Input: part model. Units: mm. Frame: model coordinates. A direction names the side the tool comes from. Round coordinates to 2 decimals unless told otherwise and drop trailing zeros. Loops run counter-clockwise (first coordinate to the right, second up) from the corner with the lowest first, then second, coordinate; pieces in that order, holes last. Notation, with made-up numbers: (16, -2) - (34, -2) arc R26 ccw to (34, 18) - close; hole circle Ø5 at (44, 14). An arc over 180 degrees is marked (long way). One line per question, with ' | ' between items. Start each with the question number.
Item 1: Set-up query: faces 4 (the face through (-7, 50, 25)), 5 (the face through (-380, 0, 25)). Return all of +Z, -Z, +X, -X, +Y, -Y with unobstructed straight access to the full face (end or side cutting, diameter ignored); none if empty.
Item 2: Material intervals for line 1 along Y through (x, z) = (60, 39); line 2 along Y through (x, z) = (-289.5, 4), sorted ascending.
Item 3: First-contact query: pin 1 (4 mm diameter, centred on x = -263, y = 16, fed in from -Z). Flat tip, straight axial feed; report the tip coordinate or a pass-through.
Item 4: Draft query along Y for faces 1 (the face through (-7, -50, 25)), 2 (the face through (-400, 10, 25)), 3 (the face through (-500, 1, 25)). Return one class per face: pulls with the +Y half, pulls with the -Y half, needs draft (parallel to the pull), parting line crosses it, or undercut.
Item 5: Section B-B, the plane y = 0. Give the number of separate pieces and of enclosed holes in the cut face, plus the area to 3 significant figures.
Item 6: Section A-A, the plane x = -392.5. Return loops of the section in (y, z), plus the area to 3 significant figures.
```python
from build123d import *

# Parameters (mm, degrees)
SKETCH1_W           = 900
SKETCH1_H           = 100
BOSS_EXTRUDE1_DEPTH = 50
SKETCH2_W           = 40
SKETCH2_H           = 20
CUT_EXTRUDE1_DEPTH  = 50
SKETCH3_W           = 50
SKETCH3_H           = 50
BOSS_EXTRUDE2_DEPTH = 100


with BuildPart() as part:
    # Sketch1 → Boss-Extrude1 (new body)
    with BuildSketch(Plane.XY):
        Rectangle(SKETCH1_W, SKETCH1_H)
    extrude(amount=BOSS_EXTRUDE1_DEPTH)

    # Sketch2 → Cut-Extrude1 (cut)
    with BuildSketch(Plane.XY.offset(50)):
        with Locations((-400, 0)):
            Rectangle(SKETCH2_W, SKETCH2_H)
        with BuildLine():
            Line((-180, 34), (-184, 34))
            Line((-184, 34), (-184, 29.732137495))
            ThreePointArc((-184, 29.732137495), (-180, -30), (-176, 29.732137495))
            Line((-176, 29.732137495), (-176, 34))
            Line((-176, 34), (-180, 34))
        make_face()
        with Locations((400, 0)):
            Rectangle(SKETCH2_W, SKETCH2_H)
        with BuildLine():
            Line((-300, 34), (-296, 34))
            Line((-296, 34), (-296, 29.732137495))
            ThreePointArc((-296, 29.732137495), (-300, -30), (-304, 29.732137495))
            Line((-304, 29.732137495), (-304, 34))
            Line((-304, 34), (-300, 34))
        make_face()
        with BuildLine():
            Line((-60, 34), (-64, 34))
            Line((-64, 34), (-64, 29.732137495))
            ThreePointArc((-64, 29.732137495), (-60, -30), (-56, 29.732137495))
            Line((-56, 29.732137495), (-56, 34))
            Line((-56, 34), (-60, 34))
        make_face()
        with BuildLine():
            Line((60, 34), (56, 34))
            Line((56, 34), (56, 29.732137495))
            ThreePointArc((56, 29.732137495), (60, -30), (64, 29.732137495))
            Line((64, 29.732137495), (64, 34))
            Line((64, 34), (60, 34))
        make_face()
        with BuildLine():
            Line((180, 34), (176, 34))
            Line((176, 34), (176, 29.732137495))
            ThreePointArc((176, 29.732137495), (180, -30), (184, 29.732137495))
            Line((184, 29.732137495), (184, 34))
            Line((184, 34), (180, 34))
        make_face()
        with BuildLine():
            Line((300, 34), (296, 34))
            Line((296, 34), (296, 29.732137495))
            ThreePointArc((296, 29.732137495), (300, -30), (304, 29.732137495))
            Line((304, 29.732137495), (304, 34))
            Line((304, 34), (300, 34))
        make_face()
    extrude(amount=-CUT_EXTRUDE1_DEPTH, mode=Mode.SUBTRACT)

    # Sketch3 → Boss-Extrude2 (add)
    with BuildSketch(Plane(origin=(0, 50, 0), x_dir=(1, 0, 0), z_dir=(0, 1, 0))):
        with Locations((475, -25)):
            Rectangle(SKETCH3_W, SKETCH3_H)
        with Locations((-475, -25)):
            Rectangle(SKETCH3_W, SKETCH3_H)
    extrude(amount=-BOSS_EXTRUDE2_DEPTH)


solid = part.part
```
Return value:
1) face 4: +Z, -Z, +X, -X, +Y | face 5: +Z, -Z
2) line 1: -50 to -30, 34 to 50 | line 2: -50 to -28.1, 28.1 to 50
3) pin 1: z = 0
4) face 1: pulls with the -Y half | face 2: undercut | face 3: needs draft
5) separate pieces: 9 | enclosed holes: 0 | area: 28,000 mm2
6) outline: (-50, 0) - (-10, 0) - (-10, 50) - (-50, 50) - close; (10, 0) - (50, 0) - (50, 50) - (10, 50) - close | area: 4,000 mm2
